Geometry: final body of the model. Coordinates: model frame, mm. A direction names the side the tool comes from. Give positions to 0.01 mm unless a question says otherwise; leave off trailing zeros. Write each loop counter-clockwise with the first axis right and the second up, starting at its lowest first coordinate (ties: lowest second). Pieces come first, ordered by that corner, then holes.
```python
from build123d import *

# Parameters (mm, degrees)
SKETCH2_R      = 3.175
EXTRUDE1_DEPTH = 6.35


with BuildPart() as part:
    # Sketch2 → Extrude1 (new body)
    with BuildSketch(Plane.XY):
        with BuildLine():
            Line((-3.877238786, 18.628018312), (-50.950345152, 9.477933344))
            ThreePointArc((-50.950345152, 9.477933344), (-53.05063868, 10.011339949), (-53.975, 11.97126639))
            Line((-53.975, 11.97126639), (-53.975, 15.24))
            Line((-53.975, 15.24), (-60.325, 15.24))
            Line((-60.325, 15.24), (-60.325, 8.89))
            Line((-60.325, 8.89), (-66.675, 8.89))
            Line((-66.675, 8.89), (-66.675, 15.24))
            Line((-66.675, 15.24), (-73.025, 15.24))
            Line((-73.025, 15.24), (-73.025, 5.08))
            ThreePointArc((-73.025, 5.08), (-72.281051224, 3.283948776), (-70.485, 2.54))
            Line((-70.485, 2.54), (70.485, 2.54))
            ThreePointArc((70.485, 2.54), (72.281051224, 3.283948776), (73.025, 5.08))
            Line((73.025, 5.08), (73.025, 15.24))
            Line((73.025, 15.24), (66.675, 15.24))
            Line((66.675, 15.24), (66.675, 8.89))
            Line((66.675, 8.89), (60.325, 8.89))
            Line((60.325, 8.89), (60.325, 15.24))
            Line((60.325, 15.24), (53.975, 15.24))
            Line((53.975, 15.24), (53.975, 11.97126639))
            ThreePointArc((53.975, 11.97126639), (53.05063868, 10.011339949), (50.950345152, 9.477933344))
            Line((50.950345152, 9.477933344), (3.877238786, 18.628018312))
            ThreePointArc((3.877238786, 18.628018312), (0, 19.001353944), (-3.877238786, 18.628018312))
        make_face()
        with Locations((0, 10.922)):
            Circle(SKETCH2_R, mode=Mode.SUBTRACT)
    extrude(amount=EXTRUDE1_DEPTH)


solid = part.part
```
Item 1: Section C-C, the plane x = -62. Return the cut outline in (y, z), plus the area to 3 significant figures.
Found:
outline: (2.54, 0) - (8.89, 0) - (8.89, 6.35) - (2.54, 6.35) - close
area: 40.3 mm2
Item 2: Pin query (flat end, axial travel): pin 1 Ø5 at (x, y) = (0, 10.922) entering from +Z; pin 2 Ø1.5 at (x, z) = (24.5, 4) entering from +Y; pin 3 Ø1.9 at (x, z) = (-56, 2) entering from +Y; pin 4 Ø1.9 at (x, z) = (62.5, 3.5) entering from +Y. Return the tip coordinate at first contact, or that it passes through.
Found:
pin 1: passes through
pin 2: stops at y = 14.77
pin 3: stops at y = 15.24
pin 4: stops at y = 8.89
Item 3: Reachability of faces 4 (the face through (-72.301, 3.304, 3.131)), 5 (the face through (-70, 15.24, 3)), 6 (the face through (-73.025, 10, 3)), 7 (the face through (70, 15.24, 3)), 8 (the face through (64, 8.89, 3)) from +Z, -Z, +X, -X, +Y, -Y: full face, straight path, thin tool, end or side. Return the list, or none.
Found:
face 4: +Z, -Z, -X, -Y
face 5: +Z, -Z, -X, +Y
face 6: +Z, -Z, -X, +Y, -Y
face 7: +Z, -Z, +X, +Y
face 8: +Z, -Z, +Y
Item 4: Pull-direction query (X, two-part tool) for faces 1 (the face through (-1, 2.54, 3)), 2 (the face through (73.025, 10, 3)), 3 (the face through (-27.084, 14.117, 3.131)); classes: +X half, -X half, draft (parallel to the pull), parting line (faces both ways), or undercut.
Found:
face 1: draft
face 2: +X half
face 3: undercut
Item 5: Section D-D, the plane x = 28. Return the cut outline in (y, z).
Found:
outline: (2.54, 0) - (13.94, 0) - (13.94, 6.35) - (2.54, 6.35) - close
Item 6: Section A-A, the plane x = 0. Return the cut outline in (y, z).
Found:
outline: (2.54, 0) - (7.75, 0) - (7.75, 6.35) - (2.54, 6.35) - close; (14.1, 0) - (19, 0) - (19, 6.35) - (14.1, 6.35) - close
Item 7: Section B-B, the plane z = 2.5. Return the cut outline in (x, y) (3 decimals).
Found:
outline: (-73.025, 5.08) arc R2.54 ccw to (-70.485, 2.54) - (70.485, 2.54) arc R2.54 ccw to (73.025, 5.08) - (73.025, 15.24) - (66.675, 15.24) - (66.675, 8.89) - (60.325, 8.89) - (60.325, 15.24) - (53.975, 15.24) - (53.975, 11.971) arc R2.54 cw to (50.95, 9.478) - (3.877, 18.628) arc R20.32 ccw to (-3.877, 18.628) - (-50.95, 9.478) arc R2.54 cw to (-53.975, 11.971) - (-53.975, 15.24) - (-60.325, 15.24) - (-60.325, 8.89) - (-66.675, 8.89) - (-66.675, 15.24) - (-73.025, 15.24) - close; hole circle Ø6.35 at (0, 10.922)
Item 8: Line query: L1, parallel to Y at x = 0, z = 4; L2, parallel to Y at x = 55, z = 5; L3, parallel to X at y = 8.5, z = 4.25 (3 decimals). Output: solid intervals per line, ascending.
Found:
L1: y = 2.54 to 7.75, 14.1 to 19
L2: y = 2.54 to 15.24
L3: x = -73.025 to -2.053, 2.053 to 73.025
